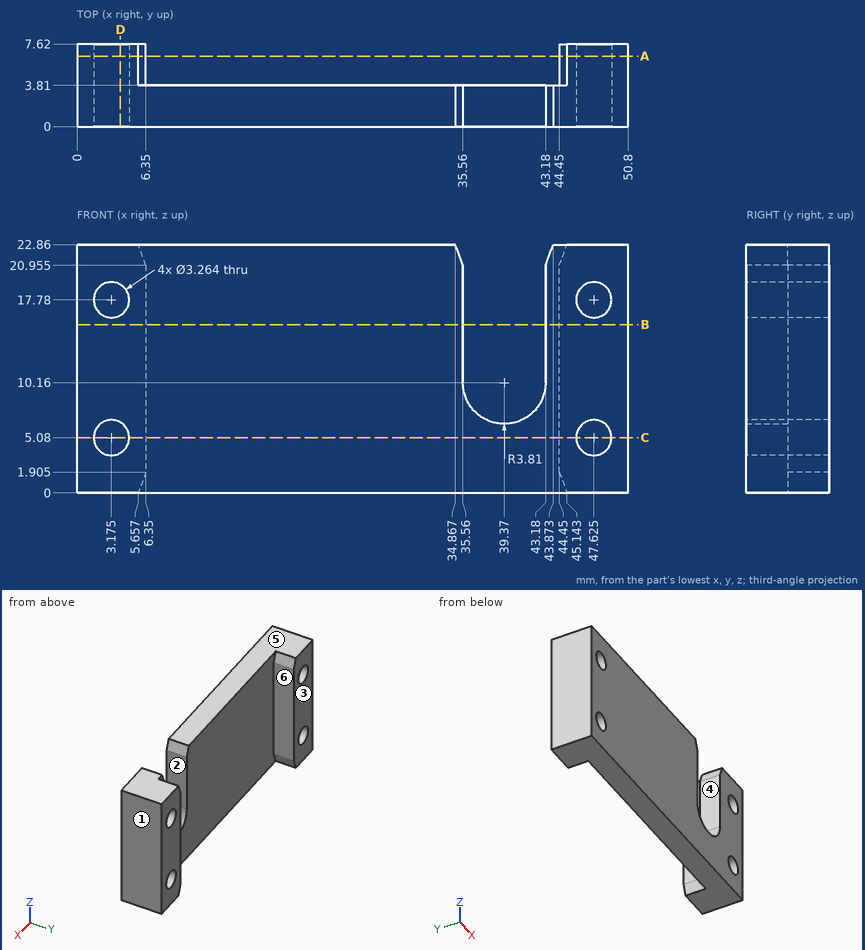
Could you check a few things on this drawing? It's one solid part, dimensions in mm from its lowest x, y, z. A direction names the side the tool comes from. Round coordinates to 2 decimals unless told otherwise and drop trailing zeros. Write each loop counter-clockwise with the first axis right and the second up, starting at its lowest first coordinate (ties: lowest second). Pieces come first, ordered by that corner, then holes.
Q1. If we section it at D-D on x = 4: Write out the boundary of the cut face in (y, z), plus the area to 3 significant figures.
Q2. If we mould it in two halves opening along X, with no side actions, what happens to the marked faces 1, 2 and 3? For each: +X half, -X half, draft (parallel to the pull), parting line (faces both ways), or undercut.
Q3. Will these pins go through, and if not, where does the flat tip stop? P1, Ø3, axis at y = 5, z = 7.5, coming from the -X side; P2, Ø2, axis at x = 3.175, z = 17.78, coming from the -Y side; P3, Ø7, axis at x = 32, z = 10.5, coming from the +Y side.
Q4. Which directions (+Z, -Z, +X, -X, +Y, -Y) give clear straight access to the entire face, cutting with the end or side of a thin tool? Please do the marked faces 4, 5 and 6.
Q5. If we section it at A-A on y = 6.5: Give the number of separate pieces and of enclosed holes in the cut face, plus the area to 3 significant figures.
Q6. Please list where these lines run through material, in increasing order: probe 1 along X at (y, z) = (6, 17.78); probe 2 along X at (y, z) = (4.25, 6); probe 3 along Z at (x, y) = (2.5, 6) (1 decimal).
Q7. If we section it at C-C on z = 5.08: Write out the boundary of the cut face in (x, y).
Q8. If we section it at B-B on z = 15.5: Write out the boundary of the cut face in (x, y), plus the area to 3 significant figures.
Answer below:
1. outline: (0, 0) - (7.62, 0) - (7.62, 3.67) - (0, 3.67) - close; (0, 6.49) - (7.62, 6.49) - (7.62, 16.37) - (0, 16.37) - close; (0, 19.19) - (7.62, 19.19) - (7.62, 22.86) - (0, 22.86) - close
1. area: 131 mm2
2. face 1: +X half
2. face 2: undercut
2. face 3: draft
3. P1: stops at x = 0
3. P2: passes through
3. P3: stops at y = 3.81
4. face 4: +Z, +Y, -Y
4. face 5: +Z, +X, -X, +Y, -Y
4. face 6: +Z, -Z, +Y
5. separate pieces: 2
5. enclosed holes: 4
5. area: 254 mm2
6. probe 1: x = 0 to 1.54, 4.81 to 6.35, 44.45 to 45.99, 49.26 to 50.8
6. probe 2: x = 0 to 1.83, 4.52 to 6.35, 44.45 to 46.28, 48.97 to 50.8
6. probe 3: z = 0 to 3.6, 6.6 to 16.3, 19.3 to 22.9
7. outline: (0, 0) - (1.54, 0) - (1.54, 7.62) - (0, 7.62) - close; (4.81, 0) - (45.99, 0) - (45.99, 7.62) - (44.45, 7.62) - (44.45, 3.81) - (6.35, 3.81) - (6.35, 7.62) - (4.81, 7.62) - close; (49.26, 0) - (50.8, 0) - (50.8, 7.62) - (49.26, 7.62) - close
8. outline: (0, 0) - (35.56, 0) - (35.56, 3.81) - (6.35, 3.81) - (6.35, 7.62) - (0, 7.62) - close; (43.18, 0) - (50.8, 0) - (50.8, 7.62) - (44.45, 7.62) - (44.45, 3.81) - (43.18, 3.81) - close
8. area: 213 mm2
